from build123d import *

# Parameters (mm, degrees)
BOSS_EXTRUDE1_DEPTH = 2.54
SKETCH3_R           = 3.3782
CUT_EXTRUDE1_DEPTH  = 130.54
SKETCH4_R           = 3.3782
CUT_EXTRUDE2_DEPTH  = 130.54


with BuildPart() as part:
    # Sketch2 → Boss-Extrude1 (new body)
    with BuildSketch(Plane.XY):
        with BuildLine():
            Line((-124.46, 25.4), (124.46, 25.4))
            ThreePointArc((124.46, 25.4), (126.256051224, 24.656051224), (127, 22.86))
            Line((127, 22.86), (127, -22.86))
            ThreePointArc((127, -22.86), (126.256051224, -24.656051224), (124.46, -25.4))
            Line((124.46, -25.4), (-124.46, -25.4))
            ThreePointArc((-124.46, -25.4), (-126.256051224, -24.656051224), (-127, -22.86))
            Line((-127, -22.86), (-127, 22.86))
            ThreePointArc((-127, 22.86), (-126.256051224, 24.656051224), (-124.46, 25.4))
        make_face()
    extrude(amount=BOSS_EXTRUDE1_DEPTH)

    # Sketch3 → Cut-Extrude1 (cut, through all)
    with BuildSketch(Plane.XY.offset(2.54)):
        with Locations((-107.95, -6.35)):
            Circle(SKETCH3_R)
    extrude(amount=-CUT_EXTRUDE1_DEPTH, mode=Mode.SUBTRACT)

    # Sketch4 → Cut-Extrude2 (cut, through all)
    with BuildSketch(Plane.XY.offset(2.54)):
        with Locations((107.95, -6.35)):
            Circle(SKETCH4_R)
    extrude(amount=-CUT_EXTRUDE2_DEPTH, mode=Mode.SUBTRACT)


solid = part.part
Build history of the part. All positions in model axes, mm. Round coordinates to 2 decimals unless told otherwise and drop trailing zeros. Write each loop counter-clockwise with the first axis right and the second up, starting at its lowest first coordinate (ties: lowest second). Pieces come first, ordered by that corner, then holes. Notation, with made-up numbers: M 58.5,-40 L 114.5,-40 A14 cw 114.5,-13 Z; hole C 68.25,58 d6. An arc over 180 degrees is marked long. Answer as a JSON object with one key per item and string values. Group by question number.
(1) Cut at A-A (x = -107.95). Give the cut face in (y, z), and give its area (3 significant figures).
(2) Mould opens along X. For faces 1 (the cylindrical face through (-105, -8, 1)), 2 (the flat face through (2, 0, 2.54)) say: pulls with the +X half, pulls with the -X half, needs draft (parallel to the pull), parting line crosses it, or undercut.
(3) Drill centre lines: L1, parallel to X at y = -4, z = 0.25; L2, parallel to X at y = -4.5, z = 0.2; L3, parallel to Y at x = -107.95, z = 1.1. Where is each one in solid material? Low to high.
(4) Cut at B-B (y = -6.35). Give the cut face in (x, z), and give its area (3 significant figures).
Responses:
{
 "1": {"outline": "M -25.4,0 L -9.73,0 L -9.73,2.54 L -25.4,2.54 Z; M -2.97,0 L 25.4,0 L 25.4,2.54 L -2.97,2.54 Z", "area": "112 mm2"},
 "2": {"face 1": "undercut", "face 2": "needs draft"},
 "3": {"L1": "x = -127 to -110.38, -105.52 to 105.52, 110.38 to 127", "L2": "x = -127 to -110.78, -105.12 to 105.12, 110.78 to 127", "L3": "y = -25.4 to -9.73, -2.97 to 25.4"},
 "4": {"outline": "M -127,0 L -111.33,0 L -111.33,2.54 L -127,2.54 Z; M -104.57,0 L 104.57,0 L 104.57,2.54 L -104.57,2.54 Z; M 111.33,0 L 127,0 L 127,2.54 L 111.33,2.54 Z", "area": "611 mm2"}
}
